from build123d import *

# Parameters (mm, degrees)
BOSS_EXTRUDE1_DEPTH = 1
SKETCH2_R           = 3.17500001
SKETCH2_R_2         = 3.175
CUT_EXTRUDE1_DEPTH  = 2
CUT_EXTRUDE2_DEPTH  = 2


with BuildPart() as part:
    # Sketch1 → Boss-Extrude1 (new body)
    with BuildSketch(Plane.XY):
        with BuildLine():
            Line((25.358256565, 64.538916848), (30.219025255, 76.273850543))
            ThreePointArc((30.219025255, 76.273850543), (-31.396114158, -75.796924606), (32.565679267, 75.301834625))
            Line((32.565679267, 75.301834625), (27.218819563, 62.393373411))
            ThreePointArc((27.218819563, 62.393373411), (-49.023820587, -47.227769363), (63.365389329, 24.872165551))
            Line((63.365389329, 24.872165551), (51.629608078, 20.011045792))
            ThreePointArc((51.629608078, 20.011045792), (-51.157057474, -21.189947017), (50.65759216, 22.357699804))
            Line((50.65759216, 22.357699804), (63.56690093, 27.704910578))
            ThreePointArc((63.56690093, 27.704910578), (-48.125948441, -49.921999666), (25.358256565, 64.538916848))
        make_face()
    extrude(amount=BOSS_EXTRUDE1_DEPTH)

    # Sketch2 → Cut-Extrude1 (cut, through all)
    with BuildSketch(Plane.XY.offset(1)):
        with Locations((61.722, 0)):
            Circle(SKETCH2_R)
        with Locations((75.692, 0)):
            Circle(SKETCH2_R_2)
        with Locations((53.522326482, -53.522326482)):
            Circle(SKETCH2_R_2)
        with Locations((43.644044748, -43.644044748)):
            Circle(SKETCH2_R)
        with Locations((0, -75.692)):
            Circle(SKETCH2_R_2)
        with Locations((0, -61.722)):
            Circle(SKETCH2_R)
        with Locations((-53.522326482, -53.522326482)):
            Circle(SKETCH2_R_2)
        with Locations((-43.644044748, -43.644044748)):
            Circle(SKETCH2_R)
        with Locations((-75.692, 0)):
            Circle(SKETCH2_R_2)
        with Locations((-61.722, 0)):
            Circle(SKETCH2_R)
        with Locations((-53.522326482, 53.522326482)):
            Circle(SKETCH2_R_2)
        with Locations((-43.644044748, 43.644044748)):
            Circle(SKETCH2_R)
        with Locations((0, 75.692)):
            Circle(SKETCH2_R_2)
        with Locations((0, 61.722)):
            Circle(SKETCH2_R)
        with Locations((53.522326482, 53.522326482)):
            Circle(SKETCH2_R_2)
        with Locations((43.644044748, 43.644044748)):
            Circle(SKETCH2_R)
    extrude(amount=-CUT_EXTRUDE1_DEPTH, mode=Mode.SUBTRACT)

    # Sketch3 → Cut-Extrude2 (cut, through all)
    with BuildSketch(Plane.XY.offset(1)):
        Polygon((61.817656075, -26.980349635), (62.990983081, -27.466357594), (63.962998999, -25.119703581), (62.789671993, -24.633695622), align=None)
        Polygon((25.119703581, -63.962998999), (27.466357594, -62.990983081), (26.980349635, -61.817656075), (24.633695622, -62.789671993), align=None)
        Polygon((-27.466357594, -62.990983081), (-25.119703581, -63.962998999), (-24.633695622, -62.789671993), (-26.980349635, -61.817656075), align=None)
        Polygon((-63.962998999, -25.119703581), (-62.990983081, -27.466357594), (-61.817656075, -26.980349635), (-62.789671993, -24.633695622), align=None)
        Polygon((-62.990983081, 27.466357594), (-63.962998999, 25.119703581), (-62.789671993, 24.633695622), (-61.817656075, 26.980349635), align=None)
        Polygon((-25.119703581, 63.962998999), (-27.466357594, 62.990983081), (-26.980349635, 61.817656075), (-24.633695622, 62.789671993), align=None)
        Polygon((27.466357594, 62.990983081), (25.119703581, 63.962998999), (24.633695622, 62.789671993), (26.980349635, 61.817656075), align=None)
        Polygon((75.696269062, 29.979783172), (76.869596069, 30.465791131), (75.89758015, 32.812445144), (74.724253144, 32.326437185), align=None)
        Polygon((75.696269062, -29.979783172), (76.869596069, -30.465791131), (75.89758015, -32.812445144), (74.724253144, -32.326437185), align=None)
        Polygon((32.326437185, -74.724253144), (32.812445144, -75.89758015), (30.465791131, -76.869596069), (29.979783172, -75.696269062), align=None)
        Polygon((-29.979783172, -75.696269062), (-30.465791131, -76.869596069), (-32.812445144, -75.89758015), (-32.326437185, -74.724253144), align=None)
        Polygon((-74.724253144, -32.326437185), (-75.89758015, -32.812445144), (-76.869596069, -30.465791131), (-75.696269062, -29.979783172), align=None)
        Polygon((-75.696269062, 29.979783172), (-76.869596069, 30.465791131), (-75.89758015, 32.812445144), (-74.724253144, 32.326437185), align=None)
        Polygon((-32.326437185, 74.724253144), (-32.812445144, 75.89758015), (-30.465791131, 76.869596069), (-29.979783172, 75.696269062), align=None)
    extrude(amount=-CUT_EXTRUDE2_DEPTH, mode=Mode.SUBTRACT)


solid = part.part
Read the model definition and answer for the solid it produces. Units are mm, in the model's axes. A direction names the side the tool comes from. Coordinates: 2 decimals unless noted, no trailing zeros. Order: outer loops, then holes, each group sorted by start corner. A loop starts at its lowest first (then second) coordinate and runs counter-clockwise, first axis right, second up. Notation, with made-up numbers: (-9.75, -14.75) -> (4.25, -14.75) arc R25 ccw to (4.25, 15.25) -> close; hole circle Ø7 at (53.5, -15). An arc over 180 degrees is marked (long way). Answer as a JSON object with one key per item and string values.
1) A tool of negligible diameter and unlimited length cuts with its end or side. For faces 1 (the face through (68.07, -0.36, 0.49)), 2 (the face through (82.04, -0.43, 0.49)), from which of +Z, -Z, +X, -X, +Y, -Y can it reach the whole face along a straight path? Write none if from no direction.
Model answer:
{"face 1": "+Z, -Z", "face 2": "+Z, -Z, +X"}
2) The mould has two halves that part along X. Classify faces 3 (the face through (-48.386, -47.881, 0.493)), 4 (the face through (-58.318, -57.705, 0.493)), 5 (the face through (54, -17, 0)): released by +X, released by -X, zero draft, split by the parting line, or undercut.
Model answer:
{"face 3": "undercut", "face 4": "released by -X", "face 5": "zero draft"}
3) Consider line 1 along X through (y, z) = (-36.5, 0.85); line 2 along X through (y, z) = (-25, 0.1); line 3 along X through (y, z) = (48.5, 0.55). Determine where each line is inside the solid, lowest interval first. Write a range as from..to.
Model answer:
{"line 1": "x = -73.48..-58.96, -57.46..-41.64, 41.64..57.46, 58.96..73.48", "line 2": "x = -78.14..-64.68, -62.64..-49.41, 49.41..62.64, 64.68..78.14", "line 3": "x = -66.17..-49.56, -47.77..-26.72, 26.72..66.17"}
4) A cutting plane is placed at C-C, the plane x = 18. Determine the outline of the cut face in (y, z).
Model answer:
{"outline": "(-80.04, 0) -> (-66.97, 0) -> (-66.97, 1) -> (-80.04, 1) -> close; (-65.65, 0) -> (-52.36, 0) -> (-52.36, 1) -> (-65.65, 1) -> close; (52.36, 0) -> (65.65, 0) -> (65.65, 1) -> (52.36, 1) -> close; (66.97, 0) -> (80.04, 0) -> (80.04, 1) -> (66.97, 1) -> close"}
5) A cutting plane is placed at A-A, the plane x = 0. State how many separate pieces and enclosed holes the cut face has, plus the area to 3 significant figures.
Model answer:
{"separate pieces": "8", "enclosed holes": "0", "area": "25.4 mm²"}
6) This flat-tipped pin is pushed along its axis until it touches: pin 1 (5 mm diameter, centred on x = -53.52, y = -53.52, fed in from +Z). Where does it stop, or does it pass through?
Model answer:
{"pin 1": "passes through"}
